Geometry: see drawing. Coordinates: mm, zero at the bounding-box minimum. Give positions to 0.01 mm unless a question says otherwise; leave off trailing zeros. Loops run counter-clockwise (first coordinate to the right, second up) from the corner with the lowest first, then second, coordinate; pieces in that order, holes last. Notation, with made-up numbers: M -4,43.25 L 48,43.25 A9 ccw 48,60.25 Z; hole C 10,66 d8. An arc over 180 degrees is marked long. Put each result on its own line as item: value.
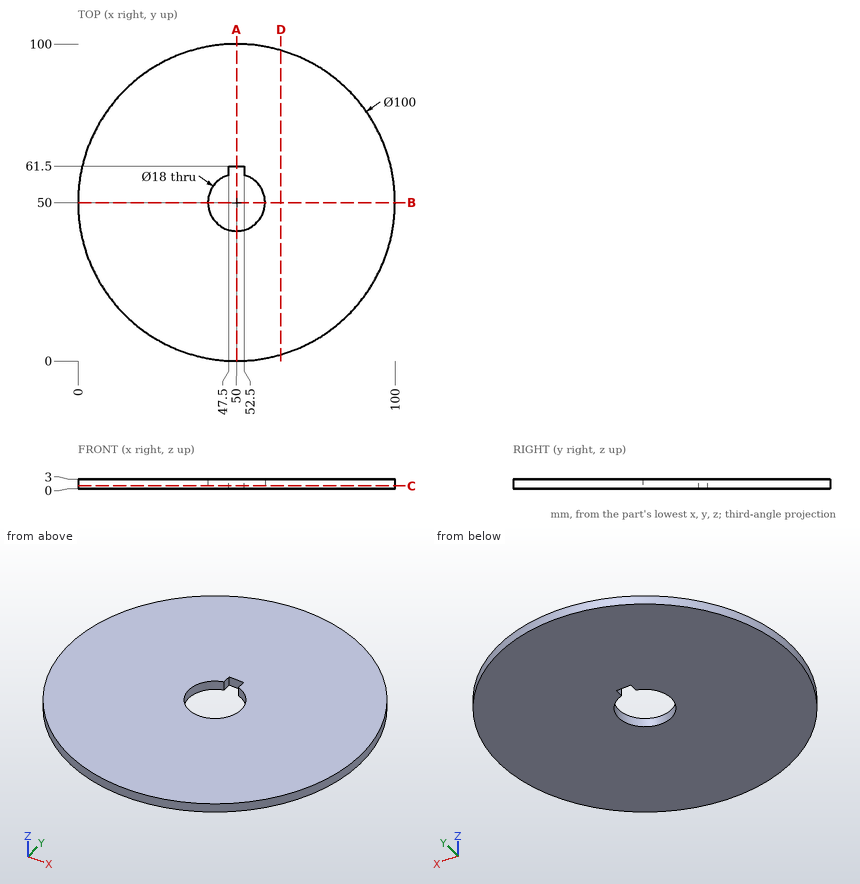
1. Contact query for flat-ended pins moving along their axis: P1, Ø0.9, axis at y = 60.5, z = 1, coming from the -X side; P2, Ø1.4, axis at y = 60.5, z = 1.5, coming from the +X side; P3, Ø1.5, axis at y = 47, z = 2, coming from the +X side. Output: stop coordinate, or through.
Found:
P1: x = 1.02
P2: x = 99.03
P3: x = 99.95
2. Section query A-A (x = 50). Output: boundary loops of the cut face in (y, z), plus the area to 4 significant figures.
Found:
outline: M 0,0 L 41,0 L 41,3 L 0,3 Z; M 61.5,0 L 100,0 L 100,3 L 61.5,3 Z
area: 238.5 mm^2
3. Section query D-D (x = 64). Output: boundary loops of the cut face in (y, z), plus the area to 3 significant figures.
Found:
outline: M 2,0 L 98,0 L 98,3 L 2,3 Z
area: 288 mm^2
4. Material intervals for line 1 (Y direction, x = 50, z = 1.2); line 2 (X direction, y = 43, z = 2.25); line 3 (X direction, y = 47, z = 2.5), sorted ascending. Write a range as from..to.
Found:
line 1: 0..41, 61.5..100
line 2: 0.49..44.34, 55.66..99.51
line 3: 0.09..41.51, 58.49..99.91
5. Section query C-C (z = 0.85). Output: boundary loops of the cut face in (x, y).
Found:
outline: C 50,50 d100; hole M 47.5,58.65 A9 ccw long 52.5,58.65 L 52.5,61.5 L 47.5,61.5 Z
6. Section query B-B (y = 50). Output: boundary loops of the cut face in (x, z).
Found:
outline: M 0,0 L 41,0 L 41,3 L 0,3 Z; M 59,0 L 100,0 L 100,3 L 59,3 Z
